```python
from build123d import *

# Parameters (mm, degrees)
SKETCH1_W                      = 50.038
SKETCH1_H                      = 50.038
SKETCH1_R                      = 20
BOSS_EXTRUDE1_DEPTH            = 20
FILLET1_R                      = 3.96875
M4X0_7_TAPPED_HOLE2_AT_2_COUNT = 2
M4X0_7_TAPPED_HOLE2_AT_2_PITCH = 30
SKETCH6_R                      = 21
SKETCH6_R_2                    = 20
BOSS_EXTRUDE2_DEPTH            = 2
FILLET2_R                      = 1


with BuildPart() as part:
    # Sketch1 → Boss-Extrude1 (new body)
    with BuildSketch(Plane.XY):
        Rectangle(SKETCH1_W, SKETCH1_H)
        Circle(SKETCH1_R, mode=Mode.SUBTRACT)
    extrude(amount=BOSS_EXTRUDE1_DEPTH)

    # Fillet1
    fillet1_edges = [part.edges().sort_by_distance(p)[0] for p in [
        (25.019, -25.019, 10),
        (-25.019, -25.019, 10),
        (-25.019, 25.019, 10),
        (25.019, 25.019, 10),
    ]]
    fillet(fillet1_edges, radius=FILLET1_R)

    # Sketch5 → M4x0.7 Tapped Hole2 (revolve, cut)
    with BuildSketch(Plane(origin=(-25.019, 15, 10), x_dir=(0, 0, 1), z_dir=(0, 1, 0))):
        Polygon((0, 0), (0, 8), (1.65, 7.008579979), (1.65, 0), align=None)
    m4x0_7_tapped_hole2 = revolve(axis=Axis((-31.369, 15, 10), (1, 0, 0)), mode=Mode.SUBTRACT)

    # M4x0.7 Tapped Hole2 at 2: M4x0.7 Tapped Hole2 ×2
    with Locations(*[(0, -i * M4X0_7_TAPPED_HOLE2_AT_2_PITCH, 0) for i in range(1, M4X0_7_TAPPED_HOLE2_AT_2_COUNT)]):
        add(m4x0_7_tapped_hole2, mode=Mode.SUBTRACT)

    # Mirror1: M4x0.7 Tapped Hole2 across plane
    add(m4x0_7_tapped_hole2.mirror(Plane(origin=(0, 0, 0), x_dir=(0, 0, 1), z_dir=(1, 0, 0))), mode=Mode.SUBTRACT)

    # Mirror1 copy 1 sketch → Mirror1 copy 1 (revolve, cut)
    with BuildSketch(Plane(origin=(25.019, -15, 10), x_dir=(0, 0, 1), z_dir=(0, 1, 0))):
        Polygon((0, 0), (0, -8), (1.65, -7.008579979), (1.65, 0), align=None)
    revolve(axis=Axis((31.369, -15, 10), (1, 0, 0)), mode=Mode.SUBTRACT)

    # Sketch6 → Boss-Extrude2 (add)
    with BuildSketch(Plane.XY.offset(20)):
        Circle(SKETCH6_R)
        Circle(SKETCH6_R_2, mode=Mode.SUBTRACT)
    extrude(amount=BOSS_EXTRUDE2_DEPTH)

    # Fillet2
    fillet2_edges = [part.edges().sort_by_distance(p)[0] for p in [
        (-21, 0, 20),
    ]]
    fillet(fillet2_edges, radius=FILLET2_R)


solid = part.part
```
Model file for the job. Use its own axes, mm. A direction names the side the tool comes from. Round coordinates to 2 decimals unless told otherwise and drop trailing zeros. Write each loop counter-clockwise with the first axis right and the second up, starting at its lowest first coordinate (ties: lowest second). Pieces come first, ordered by that corner, then holes. Notation, with made-up numbers: (-7.5, 70.5) - (11.5, 70.5) arc R19 ccw to (11.5, 98.5) - close; hole circle Ø5 at (26.5, -7). An arc over 180 degrees is marked (long way). One line per item, written item: value.
(1) Drop flat-ended pins along their axis: P1, Ø4, axis at y = 15, z = 10, coming from the -X side; P2, Ø2, axis at y = 15, z = 10, coming from the -X side; P3, Ø2.5, axis at y = -15, z = 10, coming from the -X side. Give the stop position or say it passes through.
Values follow:
P1: stops at x = -25.02
P2: stops at x = -17.62
P3: stops at x = -17.77
(2) Cut at B-B, the plane x = 0. Give the cut face in (y, z), plus the area to 3 significant figures.
Values follow:
outline: (-25.02, 0) - (-20, 0) - (-20, 22) - (-21, 22) - (-21, 21) arc R1 cw to (-22, 20) - (-25.02, 20) - close; (20, 0) - (25.02, 0) - (25.02, 20) - (22, 20) arc R1 cw to (21, 21) - (21, 22) - (20, 22) - close
area: 205 mm²
(3) Wall check: probe 1 along Y at (x, z) = (-21.25, 10); probe 2 along Y at (x, z) = (0, 17.5); probe 3 along Y at (x, z) = (-23.5, 10). Give the ranges that are in metal, low to high.
Values follow:
probe 1: y = -25.01 to -16.65, -13.35 to 13.35, 16.65 to 25.01
probe 2: y = -25.02 to -20, 20 to 25.02
probe 3: y = -24.17 to -16.65, -13.35 to 13.35, 16.65 to 24.17
(4) 3-axis set-ups, long thin cutter, end or side, ignore diameter. For faces 4 (the cylindrical face through (20.03, 6.31, 21.49)), 5 (the cylindrical face through (-21.56, -16.39, 10.89)), 6 (the cylindrical face through (21.56, 13.61, 10.89)): which of +Z, -Z, +X, -X, +Y, -Y reach the whole face in a straight line?
Values follow:
face 4: +Z
face 5: -X
face 6: +X
(5) Two-plate mould, pull along Y, no slides. Class faces 1 (the flat face through (-23, 0, 20)), 2 (the conical face through (17.19, -15.24, 10.15)), 3 (the cylindrical face through (-23.887, 23.826, 10.14)): pulls with the +Y half, pulls with the -Y half, needs draft (parallel to the pull), parting line crosses it, or undercut.
Values follow:
face 1: needs draft
face 2: undercut
face 3: pulls with the +Y half
(6) Cut at A-A, the plane z = 4. Give the cut face in (x, y), plus the area to 3 significant figures.
Values follow:
outline: (-25.02, -21.05) arc R3.97 ccw to (-21.05, -25.02) - (21.05, -25.02) arc R3.97 ccw to (25.02, -21.05) - (25.02, 21.05) arc R3.97 ccw to (21.05, 25.02) - (-21.05, 25.02) arc R3.97 ccw to (-25.02, 21.05) - close; hole circle Ø40 at (0, 0)
area: 1,230 mm²
